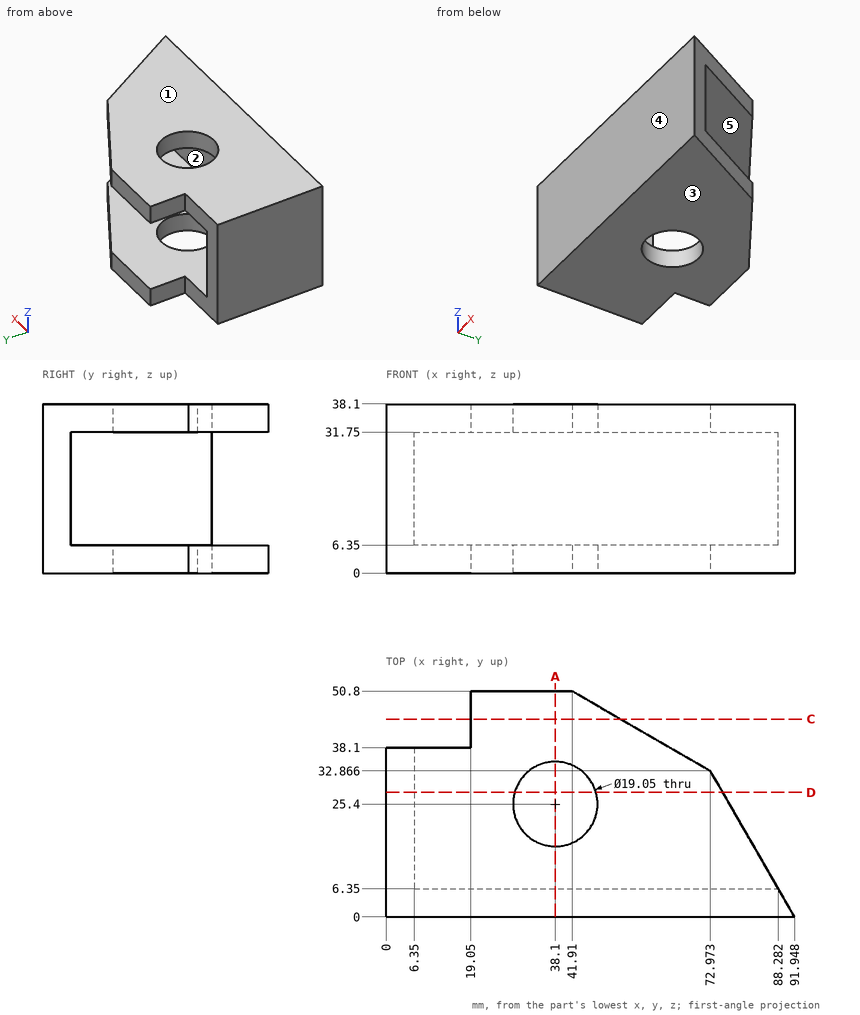
The drawing under review shows one solid part. Ordinate dimensions are in mm from its lowest x, y, z. A direction names the side the tool comes from. Round coordinates to 2 decimals unless told otherwise and drop trailing zeros. Loops run counter-clockwise (first coordinate to the right, second up) from the corner with the lowest first, then second, coordinate; pieces in that order, holes last. Notation, with made-up numbers: (53.5, 68.25) - (58.5, 68.25) arc R25 ccw to (58.5, 90.25) - close; hole circle Ø1 at (80.5, 4). An arc over 180 degrees is marked (long way). One line per item, written item: value. Start each with the question number.
1) For the marked faces 4 and 5, list the 3-axis set-ups (+Z, -Z, +X, -X, +Y, -Y) from which the entire face can be reached by the end or side of a thin tool; tool diameter is ignored.
2) Insertion check: pin 1 Ø20.5 at (y, z) = (30, 13) entering from +X; pin 2 Ø8 at (x, z) = (60, 8.5) entering from +Y; pin 3 Ø7 at (y, z) = (43.5, 3.5) entering from -X. Each pin has a flat end and moves straight along its axis. Give the tip position at first contact, or say it passes through.
3) Consider section A-A on x = 38.1. Give the boundary of the cut face in (y, z) (3 decimals).
4) Consider section C-C on y = 44.5. Give the boundary of the cut face in (x, z).
5) Consider section D-D on y = 28. Give the boundary of the cut face in (x, z), then the cut area to 3 significant figures.
6) To check wall thickness, follow L1, parallel to Z at x = 75.5, y = 18; L2, parallel to Y at x = 38.1, z = 36.25 (3 decimals); L3, parallel to Y at x = 80.5, z = 22. State the ranges of each line that lie inside material, in increasing order. Write a range as from..to.
7) Draft analysis for pull direction Z (two halves, no side actions). For the marked faces 1, 2 and 3, state which applies: +Z half, -Z half, draft (parallel to the pull), parting line (faces both ways), or undercut.
Reported:
1. face 4: +Z, -Z, +X, -X, -Y
1. face 5: +X, +Y
2. pin 1: stops at x = 79.13
2. pin 2: stops at y = 42.3
2. pin 3: stops at x = 19.05
3. outline: (0, 0) - (15.875, 0) - (15.875, 6.35) - (6.35, 6.35) - (6.35, 31.75) - (15.875, 31.75) - (15.875, 38.1) - (0, 38.1) - close; (34.925, 0) - (50.8, 0) - (50.8, 6.35) - (34.925, 6.35) - close; (34.925, 31.75) - (50.8, 31.75) - (50.8, 38.1) - (34.925, 38.1) - close
4. outline: (19.05, 0) - (52.82, 0) - (52.82, 6.35) - (19.05, 6.35) - close; (19.05, 31.75) - (52.82, 31.75) - (52.82, 38.1) - (19.05, 38.1) - close
5. outline: (0, 0) - (28.94, 0) - (28.94, 6.35) - (6.35, 6.35) - (6.35, 31.75) - (28.94, 31.75) - (28.94, 38.1) - (0, 38.1) - close; (47.26, 0) - (75.78, 0) - (75.78, 6.35) - (47.26, 6.35) - close; (47.26, 31.75) - (75.78, 31.75) - (75.78, 38.1) - (47.26, 38.1) - close
5. area: 891 mm^2
6. L1: z = 0..6.35, 31.75..38.1
6. L2: y = 0..15.875, 34.925..50.8
6. L3: y = 0..6.35
7. face 1: +Z half
7. face 2: undercut
7. face 3: -Z half
